```python
from build123d import *
from build123d.topology import SkipClean

# Parameters (mm, degrees)
EXTRUDE_2_DEPTH          = 4.5
EXTRUDE_2_DEPTH_BACK     = 4.5
CUT_EXTRUDE_1_DEPTH      = 7
CUT_EXTRUDE_1_DEPTH_BACK = 6
CUT_EXTRUDE_2_DEPTH      = 6
CUT_EXTRUDE_2_DEPTH_BACK = 6
SKETCH_10_R              = 2.2
CUT_EXTRUDE_3_DEPTH      = 2.5
SKETCH_13_R              = 3.5
SKETCH_13_R_2            = 2.2
EXTRUDE_3_DEPTH          = 2
CHAMFER_3_SIZE           = 0.5
SKETCH_18_R              = 5
EXTRUDE_5_DEPTH          = 6
SKETCH_19_R              = 4
CUT_EXTRUDE_5_DEPTH      = 16
CHAMFER_4_SIZE           = 1
SKETCH_22_R              = 1.5
CUT_EXTRUDE_6_DEPTH      = 10


with BuildPart() as part:
    # 草图5 → 凸台-拉伸2 (new, two sides: drawn at the far end of the back side and taken through both)
    with BuildSketch(Plane(origin=(0, 0, 0), x_dir=(0, 0, -1), z_dir=(1, 0, 0)).offset(-EXTRUDE_2_DEPTH_BACK)):
        with BuildLine():
            Line((0, -6), (18, -6))
            ThreePointArc((18, -6), (24, 0), (18, 6))
            Line((18, 6), (0, 6))
            ThreePointArc((0, 6), (-6, 0), (0, -6))
        make_face()
    extrude(amount=EXTRUDE_2_DEPTH + EXTRUDE_2_DEPTH_BACK)

    # 草图7 → 切除-拉伸1 (cut, two sides: drawn at the far end of the back side and taken through both)
    with BuildSketch(Plane(origin=(0, 0, 0), x_dir=(0, 0, -1), z_dir=(1, 0, 0)).offset(-CUT_EXTRUDE_1_DEPTH_BACK)):
        with BuildLine():
            ThreePointArc((3.464101615, 2), (-4, 0), (3.464101615, -2))
            ThreePointArc((3.464101615, -2), (4, 0), (3.464101615, 2))
        make_face()
    extrude(amount=CUT_EXTRUDE_1_DEPTH + CUT_EXTRUDE_1_DEPTH_BACK, mode=Mode.SUBTRACT)

    # 草图10 → 切除-拉伸2 (cut, two sides: drawn at the far end of the back side and taken through both)
    with BuildSketch(Plane(origin=(0, 0, 0), x_dir=(0, 0, -1), z_dir=(1, 0, 0)).offset(-CUT_EXTRUDE_2_DEPTH_BACK)):
        with Locations((18, 0)):
            Circle(SKETCH_10_R)
    extrude(amount=CUT_EXTRUDE_2_DEPTH + CUT_EXTRUDE_2_DEPTH_BACK, mode=Mode.SUBTRACT)

    # 草图11 → 切除-拉伸3 (cut)
    with BuildSketch(Plane.ZY.offset(4.5)):
        with BuildLine():
            Line((-18, 6), (0, 6))
            ThreePointArc((0, 6), (-6, 0), (0, -6))
            Line((0, -6), (-18, -6))
            ThreePointArc((-18, -6), (-24, 0), (-18, 6))
        make_face()
    cut_extrude_3 = extrude(amount=-CUT_EXTRUDE_3_DEPTH, mode=Mode.SUBTRACT)

    # 镜向2: 切除-拉伸3 across plane
    add(cut_extrude_3.mirror(Plane(origin=(0, 0, 0), x_dir=(0, 0, 1), z_dir=(1, 0, 0))), mode=Mode.SUBTRACT)

    # 草图13 → 凸台-拉伸3 (add)
    with SkipClean():  # the faces are left unmerged after this step: merging them gives an invalid solid
        with BuildSketch(Plane.ZY.offset(2)):
            with Locations((-18, 0)):
                Circle(SKETCH_13_R)
            with Locations((-18, 0)):
                Circle(SKETCH_13_R_2, mode=Mode.SUBTRACT)
        extrude(amount=EXTRUDE_3_DEPTH)

    # 倒角3
    chamfer_3_edges = [part.edges().sort_by_distance(p)[0] for p in [
        (-4, 0, -21.5),
    ]]
    chamfer(chamfer_3_edges, length=CHAMFER_3_SIZE)

    # 草图18 → 凸台-拉伸5 (add)
    with SkipClean():  # the faces are left unmerged after this step: merging them gives an invalid solid
        with BuildSketch(Plane(origin=(4.5, 0, 0), x_dir=(0, 0, -1), z_dir=(1, 0, 0))):
            Circle(SKETCH_18_R)
        extrude(amount=EXTRUDE_5_DEPTH)

    # 草图19 → 切除-拉伸5 (cut)
    with SkipClean():  # the faces are left unmerged after this step: merging them gives an invalid solid
        with BuildSketch(Plane(origin=(10.5, 0, 0), x_dir=(0, 0, -1), z_dir=(1, 0, 0))):
            Circle(SKETCH_19_R)
        extrude(amount=-CUT_EXTRUDE_5_DEPTH, mode=Mode.SUBTRACT)

    # 倒角4
    chamfer_4_edges = [part.edges().sort_by_distance(p)[0] for p in [
        (-4.5, -1.03527618, -3.863703305),
    ]]
    chamfer(chamfer_4_edges, length=CHAMFER_4_SIZE)

    # 草图22 → 切除-拉伸6 (cut)
    with SkipClean():  # the faces are left unmerged after this step: merging them gives an invalid solid
        with BuildSketch(Plane.XY.offset(6)):
            Circle(SKETCH_22_R)
        extrude(amount=-CUT_EXTRUDE_6_DEPTH, mode=Mode.SUBTRACT)


solid = part.part
```
Check sheet for the modelled part. Datum: model origin and axes. Units: mm. A direction names the side the tool comes from. Coordinates: 2 decimals unless noted, no trailing zeros. Loops run counter-clockwise (first coordinate to the right, second up) from the corner with the lowest first, then second, coordinate; pieces in that order, holes last.
1) Sectioned sample at B-B (z = -9). Record the boundary of the cut face in (x, y), and give its area (3 significant figures).
2) Access from +Z, -Z, +X, -X, +Y, -Y to the whole of each face (thin tool, end or side, straight path). Record for faces 1 (the face through (-4, 2, -20)), 2 (the face through (-0.325, -1.464, 4.87)), 3 (the face through (-0.063, 3.226, 5.059)), 4 (the face through (4.5, 4, 4)).
3) Sectioned sample at C-C (x = 3). Record the boundary of the cut face in (y, z), and give its area (3 significant figures).
4) Gauge pin test, flat ends, axial feed: pin 1 (3 mm diameter, centred on x = 0.5, y = 4.5, fed in from -Z); pin 2 (2 mm diameter, centred on y = -2.5, z = -14, fed in from +X); pin 3 (0.5 mm diameter, centred on x = -0.5, y = -0.5, fed in from +Z); pin 4 (4 mm diameter, centred on x = 1, y = -2, fed in from -Z). Record the tip position at first contact, or that the pin passes through.
5) Material ranges on probe 1 along Y at (x, z) = (0.7, -18); probe 2 along Z at (x, y) = (1.75, -0.25); probe 3 along Z at (x, y) = (2.25, 0), recorded low to high.
6) Sectioned sample at A-A (x = 0). Record the boundary of the cut face in (y, z).
7) Release check for a two-part mould opening along Z. For faces 5 (the face through (-2.74, 1.05, -14.66)), 6 (the face through (7.46, -4.88, 1.08)), 7 (the face through (0, 6, -9)), 8 (the face through (-2, 0, -12)) record: released by +Z, released by -Z, zero draft, split by the parting line, or undercut.
8) Sectioned sample at D-D (x = 8). Record the boundary of the cut face in (y, z).
Check sheet entries:
1. outline: (-2, -6) - (2, -6) - (2, 6) - (-2, 6) - close
1. area: 48.0 mm2
2. face 1: -Z, -X, +Y, -Y
2. face 2: +Z
2. face 3: none
2. face 4: +X
3. outline: circle Ø12 at (0, 0); hole circle Ø8 at (0, 0)
3. area: 62.8 mm2
4. pin 1: stops at z = -23.2
4. pin 2: stops at x = 2
4. pin 3: stops at z = -4
4. pin 4: stops at z = -24
5. probe 1: y = -6 to -2.2, 2.2 to 6
5. probe 2: z = -23.99 to -20.19, -15.81 to -3.99, 3.99 to 5.99
5. probe 3: z = -6 to -4, 4 to 6
6. outline: (-6, -18) arc R6 ccw to (6, -18) - (6, 0) arc R6 ccw to (1.5, 5.81) - (1.5, 3.71) arc R4 cw to (1.5, -3.71) - (1.5, -4) - (-1.5, -4) - (-1.5, -3.71) arc R4 cw to (-1.5, 3.71) - (-1.5, 5.81) arc R6 ccw to (-6, 0) - close; hole circle Ø4.4 at (0, -18)
7. face 5: undercut
7. face 6: split by the parting line
7. face 7: zero draft
7. face 8: undercut
8. outline: circle Ø10 at (0, 0); hole circle Ø8 at (0, 0)
